```python
from build123d import *

# Parameters (mm, degrees)
F0_W     = 152.4
F0_H     = 127
F0_R     = 44.45
F1_DEPTH = 6.35
F4_D     = 3.7973
F6_D     = 4.4958


with BuildPart() as f1:
    # F0 (on Front) → F1 (new body)
    with BuildSketch(Plane.XZ):
        Rectangle(F0_W, F0_H)
        Circle(F0_R, mode=Mode.SUBTRACT)
    extrude(amount=F1_DEPTH)

    # F4 (through all)
    with Locations(Plane(origin=(0, 0, 0), x_dir=(-1, 0, 0), z_dir=(0, 1, 0))):
        with Locations((-60.325, 0), (0, 53.975), (60.325, 0), (0, -53.975)):
            Hole(F4_D / 2)

    # F6 (through all)
    with Locations(Plane.XZ.offset(6.35)):
        with Locations((-60.96, -44.45), (60.96, -44.45)):
            Hole(F6_D / 2)


solid = f1.part
```
Input: part model. Units: mm. Frame: model coordinates. Give positions to 0.01 mm unless a question says otherwise; leave off trailing zeros. Write each loop counter-clockwise with the first axis right and the second up, starting at its lowest first coordinate (ties: lowest second). Pieces come first, ordered by that corner, then holes. Notation, with made-up numbers: (30, -32.5) - (34, -32.5) arc R13 ccw to (34, -27.5) - close; hole circle Ø1 at (-3.75, 10). An arc over 180 degrees is marked (long way). Write item = value, one per line. Start each with the question number.
1. Section query A-A, the plane x = 0. Output: boundary loops of the cut face in (y, z), then the cut area to 3 significant figures.
2. First-contact query: pin 1 Ø2.5 at (x, z) = (0, 53.975) entering from -Y. Flat tip, straight axial feed; report the tip coordinate or a pass-through.
3. Ray query, L1, parallel to Z at x = 0, y = -1.25; L2, parallel to Z at x = -1, y = -1.25; L3, parallel to Z at x = 60.96, y = -3.5. Return the intervals inside material, ascending.
4. Section query D-D, the plane y = -2.25. Output: boundary loops of the cut face in (x, z) (3 decimals), then the cut area to 3 significant figures.
5. Section query B-B, the plane z = 0. Output: boundary loops of the cut face in (x, y), then the cut area to 3 significant figures.
6. Section query C-C, the plane z = -24.5. Output: boundary loops of the cut face in (x, y).
7. Mould query, pull axis X, two halves, no side actions, for faces 1 (the cylindrical face through (58.43, -3.22, 0.08)), 2 (the flat face through (76.2, -3, -1)), 3 (the flat face through (-76.2, -3, -1)), 4 (the cylindrical face through (-0.41, -3.22, -55.83)). Classes: released by +X, released by -X, zero draft, split by the parting line, or undercut.
Check sheet entries:
q1.outline = (-6.35, -63.5) - (0, -63.5) - (0, -55.87) - (-6.35, -55.87) - close; (-6.35, -52.08) - (0, -52.08) - (0, -44.45) - (-6.35, -44.45) - close; (-6.35, 44.45) - (0, 44.45) - (0, 52.08) - (-6.35, 52.08) - close; (-6.35, 55.87) - (0, 55.87) - (0, 63.5) - (-6.35, 63.5) - close
q1.area = 194 mm2
q2.pin_1 = through
q3.L1 = -63.5 to -55.87, -52.08 to -44.45, 44.45 to 52.08, 55.87 to 63.5
q3.L2 = -63.5 to -55.59, -52.36 to -44.44, 44.44 to 52.36, 55.59 to 63.5
q3.L3 = -63.5 to -46.7, -42.2 to -1.79, 1.79 to 63.5
q4.outline = (-76.2, -63.5) - (76.2, -63.5) - (76.2, 63.5) - (-76.2, 63.5) - close; hole circle Ø4.496 at (-60.96, -44.45); hole circle Ø3.797 at (-60.325, 0); hole circle Ø88.9 at (0, 0); hole circle Ø3.797 at (0, -53.975); hole circle Ø3.797 at (0, 53.975); hole circle Ø3.797 at (60.325, 0); hole circle Ø4.496 at (60.96, -44.45)
q4.area = 13,100 mm2
q5.outline = (-76.2, -6.35) - (-62.22, -6.35) - (-62.22, 0) - (-76.2, 0) - close; (-58.43, -6.35) - (-44.45, -6.35) - (-44.45, 0) - (-58.43, 0) - close; (44.45, -6.35) - (58.43, -6.35) - (58.43, 0) - (44.45, 0) - close; (62.22, -6.35) - (76.2, -6.35) - (76.2, 0) - (62.22, 0) - close
q5.area = 355 mm2
q6.outline = (-76.2, -6.35) - (-37.09, -6.35) - (-37.09, 0) - (-76.2, 0) - close; (37.09, -6.35) - (76.2, -6.35) - (76.2, 0) - (37.09, 0) - close
q7.face_1 = undercut
q7.face_2 = released by +X
q7.face_3 = released by -X
q7.face_4 = undercut
